Build history of the part. All positions in model axes, mm. Face numbers are marked on the shaded views. A direction names the side the tool comes from. Coordinates: 2 decimals unless noted, no trailing zeros. Order: outer loops, then holes, each group sorted by start corner. A loop starts at its lowest first (then second) coordinate and runs counter-clockwise, first axis right, second up. Notation, with made-up numbers: M -39.5,57.25 L 11.5,57.25 A14 ccw 11.5,65.25 Z; hole C 50,43 d8. An arc over 180 degrees is marked long. Use a Markdown table: item, result. Add a question column.
Autodesk Inventor part; units mm, degrees
ref_plane "YZ Plane" through (0, 0, 0) normal (1, 0, 0) x (0, 1, 0)
ref_plane "XZ Plane" through (0, 0, 0) normal (0, 1, 0) x (-1, 0, 0)
ref_plane "XY Plane" through (0, 0, 0) normal (0, 0, 1) x (1, 0, 0)
sketch "Sketch1" plane through (0, 0, 0) normal (0, 1, 0) x (-1, 0, 0)
  circle A0 centre (0, 0) radius 4
  dimension "d0" = 8
extrude "Extrusion1" add sketch "Sketch1" along normal blind 45
sketch "Sketch2" plane through (0, 45, 0) normal (0, 1, 0) x (1, 0, 0)
  circle A0 centre (0, 0) radius 4
extrude "Extrusion2" add sketch "Sketch2" along normal blind 5 draft 5
sketch "Sketch3" plane through (0, 50, 0) normal (0, 1, 0) x (1, 0, 0)
  circle A0 centre (0, 0) radius 4.4374
extrude "Extrusion3" add sketch "Sketch3" along normal blind 10
chamfer "Chamfer1" distance 1 angle 45 1 edges at (-4.4374, 60, 0)
properties part number "Handbar"
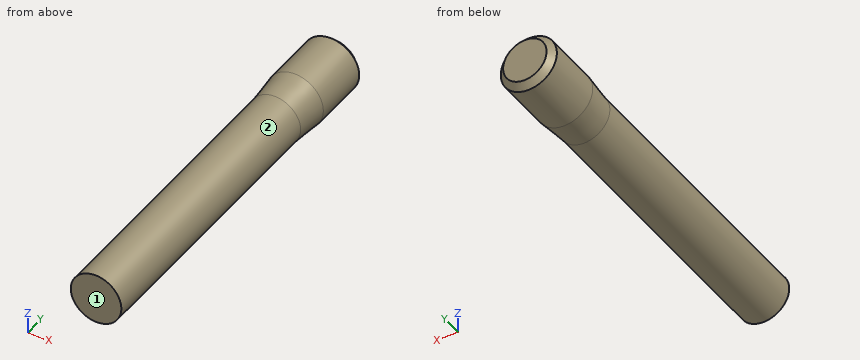
(1) Drill centre lines: line 1 along X through (y, z) = (37.5, 0); line 2 along X through (y, z) = (46.5, 2.25); line 3 along Z through (x, y) = (-2.5, 30). Where is each one in solid material? Low to high. Write a range as from..to.
(2) Slice it at D-D on y = 17.5. Give the cut face in (x, z), and give its area (3 significant figures).
(3) Drop flat-ended pins along their axis: P1, Ø1, axis at x = -1, y = 7.5, coming from the +Z side; P2, Ø1, axis at y = 23, z = 1, coming from the -X side; P3, Ø1.5, axis at y = 44.5, z = 3, coming from the +X side. Give the stop position or say it passes through.
(4) Slice it at C-C on y = 54. Give the cut face in (x, z), and give its area (3 significant figures).
(5) Which spindle directions (+Z, -Z, +X, -X, +Y, -Y) get a long thin tool onto all of the face, cutting with end or side? Do the marked faces 1 and 2. Say none if no direction does.
Solutions:
| question | item | result |
|---|---|---|
| 1 | line 1 | -4..4 |
| 1 | line 2 | -3.46..3.46 |
| 1 | line 3 | -3.12..3.12 |
| 2 | outline | C 0,0 d8 |
| 2 | area | 50.3 mm² |
| 3 | P1 | z = 3.97 |
| 3 | P2 | x = -3.97 |
| 3 | P3 | x = 3.31 |
| 4 | outline | C 0,0 d8.87 |
| 4 | area | 61.9 mm² |
| 5 | face 1 | +Z, -Z, +X, -X, -Y |
| 5 | face 2 | -Y |
